Autodesk Inventor part; units mm, degrees
ref_plane "YZ Plane" through (0, 0, 0) normal (1, 0, 0) x (0, 1, 0)
ref_plane "XZ Plane" through (0, 0, 0) normal (0, 1, 0) x (-1, 0, 0)
sketch "Sketch10" plane through (0, 0, 0) normal (0, 1, 0) x (-1, 0, 0)
  line L0 (88.9, 58.7375) -> (-88.9, 58.7375)
  line L1 (-88.9, 58.7375) -> (-88.9, -58.7375)
  line L2 (-88.9, -58.7375) -> (88.9, -58.7375)
  line L3 (88.9, -58.7375) -> (88.9, 58.7375)
  line L4 (88.9, 58.7375) -> (-88.9, -58.7375) construction
  line L5 (-88.9, 58.7375) -> (88.9, -58.7375) construction
  circle A0 centre (0, 0) radius 22.86
  dimension "d56" = 177.8
  dimension "d57" = 45.72
extrude "Extrusion5" add sketch "Sketch10" against normal blind 12.7
sketch "Sketch11" plane through (0, 0, 0) normal (0, 1, 0) x (1, 0, 0)
  point P0 (0, 0)
  point P1 (0, 31.75)
  dimension "d60" = 31.75
hole "Hole4" at (0, 0, -31.75) direction (0, -1, 0) diameter 2.6416 end through all counterbore diameter 4.699 counterbore depth 7.1374
pattern_circular "Circular Pattern1" count 6 over 360 about axis through (0, -10, 0) along (0, 1, 0) of "Hole4"
sketch "Sketch12" plane through (0, 0, 0) normal (0, 1, 0) x (1, 0, 0)
  line L0 (-88.9, -58.7375) -> (-88.9, 58.7375)
  line L1 (-88.9, 58.7375) -> (-38.1, 58.7375)
  line L2 (-38.1, 58.7375) -> (-38.1, 46.0375)
  line L3 (-38.1, 46.0375) -> (-88.9, 46.0375)
  line L4 (-88.9, 46.0375) -> (-88.9, 58.7375)
  point P0 (0, 0)
  dimension "d71" = 12.7
  dimension "d72" = 50.8
extrude "Extrusion6" add sketch "Sketch12" along normal blind 12.7
mirror "Mirror2" about plane through (0, 0, 0) normal (0, 0, 1) of "Extrusion6"
sketch "Sketch13" plane through (88.9, -12.7, -58.7375) normal (0, 0, -1) x (-1, 0, 0)
  line L0 (127, 25.4) -> (177.8, 25.4)
  circle A0 centre (147.6375, 25.4) radius 6.604
  point P0 (88.9, 12.7)
  dimension "d75" = 13.208
extrude "Extrusion7" cut sketch "Sketch13" against normal through all
sketch "Sketch14" plane through (0, 0, 0) normal (0, 1, 0) x (1, 0, 0)
  line L0 (-88.9, 46.0375) -> (-76.2, 46.0375)
  line L1 (-76.2, 46.0375) -> (-76.2, -46.0375)
  line L2 (-76.2, -46.0375) -> (-88.9, -46.0375)
  line L3 (-88.9, -46.0375) -> (-88.9, 46.0375)
  point P0 (0, 0)
  dimension "d78" = 12.7
extrude "Extrusion8" add sketch "Sketch14" along normal blind 25.4
sketch "Sketch15" plane through (0, 0, 0) normal (0, 1, 0) x (1, 0, 0)
  line L0 (88.9, 58.7375) -> (-38.1, 58.7375)
  line L1 (-38.1, -58.7375) -> (88.9, -58.7375)
  line L2 (57.15, 58.7375) -> (69.85, 58.7375)
  line L3 (69.85, 58.7375) -> (69.85, -58.7375)
  line L4 (69.85, -58.7375) -> (57.15, -58.7375)
  line L5 (57.15, -58.7375) -> (57.15, 58.7375)
  line L6 (-88.9, 46.0375) -> (-88.9, -46.0375)
  point P0 (0, 0)
  dimension "d81" = 12.7
  dimension "d82" = 146.05
extrude "Extrusion9" add sketch "Sketch15" along normal blind 25.4
sketch "Sketch16" plane through (0, 0, 0) normal (0, 1, 0) x (1, 0, 0)
  line L0 (88.9, 58.7375) -> (69.85, 58.7375)
  line L1 (88.9, -58.7375) -> (69.85, -58.7375)
  line L2 (69.85, -58.7375) -> (69.85, 58.7375)
  line L3 (69.85, 58.7375) -> (88.9, 58.7375)
  line L4 (88.9, 58.7375) -> (88.9, -58.7375)
  point P0 (0, 0)
extrude "Extrusion10" cut sketch "Sketch16" against normal through all
sketch "Sketch18" plane through (0, -12.7, 0) normal (0, -1, 0) x (1, 0, 0)
  line L0 (-88.9, 58.7375) -> (-88.9, 46.0375) construction
  line L1 (-88.9, 52.3875) -> (69.85, 52.3875) construction
  line L2 (69.85, 58.7375) -> (69.85, -58.7375) construction
  line L3 (-88.9, -58.7375) -> (-88.9, -46.0375) construction
  line L4 (-88.9, -52.3875) -> (69.85, -52.3875) construction
  line L5 (-65.3415, -46.0375) -> (-65.3415, -58.7375)
  line L6 (-65.3415, -58.7375) -> (-88.9, -58.7375)
  line L7 (-88.9, -58.7375) -> (-88.9, -46.0375)
  line L8 (-88.9, -46.0375) -> (-76.2, -46.0375)
  line L9 (-76.2, -46.0375) -> (-65.3415, -46.0375)
  line L10 (-52.1335, -58.7375) -> (-52.1335, -46.0375)
  line L11 (-52.1335, -46.0375) -> (-38.1, -46.0375)
  line L12 (-38.1, -46.0375) -> (-38.1, -58.7375)
  line L13 (-38.1, -58.7375) -> (-52.1335, -58.7375)
  line L14 (-88.9, 58.7375) -> (-88.9, -58.7375)
  line L15 (-88.9, 0) -> (69.85, 0) construction
  line L16 (69.85, -58.7375) -> (69.85, 58.7375) construction
  point P0 (0, 0)
  point P1 (-79.375, -52.3875)
  point P2 (-47.625, -52.3875)
  point P3 (-79.375, 52.3875)
  point P4 (-47.625, 52.3875)
  dimension "d94" = 9.525
  dimension "d95" = 9.525
hole "Hole6" at (-79.375, -12.7, -52.3875) at (-47.625, -12.7, -52.3875) at (-79.375, -12.7, 52.3875) at (-47.625, -12.7, 52.3875) direction (0, 1, 0) diameter 3.81 end through all
sketch "Sketch19" plane through (0, 0, 0) normal (0, 1, 0) x (1, 0, 0)
  line L0 (-74.6125, 31.75) -> (-74.6125, -31.75)
  line L1 (-74.6125, -31.75) -> (-46.0375, -31.75)
  line L2 (-46.0375, -31.75) -> (-46.0375, 31.75)
  line L3 (-46.0375, 31.75) -> (-74.6125, 31.75)
  line L4 (-74.6125, 31.75) -> (-46.0375, -31.75) construction
  line L5 (-74.6125, -31.75) -> (-46.0375, 31.75) construction
  point P0 (0, 0)
  point P1 (-60.325, 0)
extrude "Extrusion11" cut sketch "Sketch19" against normal blind 12.7
equation "\"length\" = 69.0372"
properties part number "SupportForAxel" material "PBT Plastic"
Part model, mm, in its own coordinate system. A direction names the side the tool comes from. Round coordinates to 2 decimals unless told otherwise and drop trailing zeros. Loops run counter-clockwise (first coordinate to the right, second up) from the corner with the lowest first, then second, coordinate; pieces in that order, holes last.
1. 3-axis set-ups, long thin cutter, end or side, ignore diameter. For faces 3 (the face through (-61, -6, 31.75)), 4 (the face through (-77, 12.7, -52)), 5 (the face through (-58.592, 6.098, 52.299)), 6 (the face through (-0.71, -3.62, -29.51)), 7 (the face through (-45, 12.7, 52)): which of +Z, -Z, +X, -X, +Y, -Y reach the whole face in a straight line?
Solutions:
face 3: +Y, -Y
face 4: -Z, -X, +Y
face 5: +Z, -Z, +Y
face 6: +Y
face 7: +Z, -Z, -X, +Y
2. Slice it at B-B (y = 16.5). Give the cut face in (x, z).
Solutions:
outline: (-88.9, -46.04) - (-76.2, -46.04) - (-76.2, 46.04) - (-88.9, 46.04) - close; (57.15, -58.74) - (69.85, -58.74) - (69.85, 58.74) - (57.15, 58.74) - close
3. Slice it at C-C (x = -70). Give the cut face in (y, z), and give its area (3 significant figures).
Solutions:
outline: (-12.7, -58.74) - (12.7, -58.74) - (12.7, -46.04) - (0, -46.04) - (0, -31.75) - (-12.7, -31.75) - close; (-12.7, 31.75) - (0, 31.75) - (0, 46.04) - (12.7, 46.04) - (12.7, 58.74) - (-12.7, 58.74) - close
area: 1,010 mm2
4. Flat gauge pins, fed straight in: pin 1 (6 mm diameter, centred on x = -47.62, z = 52.39, fed in from +Y); pin 2 (7.5 mm diameter, centred on x = 27.5, z = 15.88, fed in from +Y); pin 3 (3 mm diameter, centred on x = 0, z = -31.75, fed in from +Y). Where does each tip first touch, or does it go through?
Solutions:
pin 1: stops at y = 12.7
pin 2: stops at y = 0
pin 3: stops at y = -7.14
5. Two-plate mould, pull along Z, no slides. Class faces 1 (the face through (57.15, 13, 1)), 2 (the face through (-46.038, -6, 0)): pulls with the +Z half, pulls with the -Z half, needs draft (parallel to the pull), parting line crosses it, or undercut.
Solutions:
face 1: needs draft
face 2: undercut
6. Slice it at A-A (z = 0). Give the cut face in (x, y), and give its area (3 significant figures).
Solutions:
outline: (-88.9, -12.7) - (-74.61, -12.7) - (-74.61, 0) - (-76.2, 0) - (-76.2, 25.4) - (-88.9, 25.4) - close; (-46.04, -12.7) - (-22.86, -12.7) - (-22.86, 0) - (-46.04, 0) - close; (22.86, -12.7) - (69.85, -12.7) - (69.85, 25.4) - (57.15, 25.4) - (57.15, 0) - (22.86, 0) - close
area: 1,720 mm2
7. Slice it at D-D (y = -5). Count the separate pieces of the cut face and the enclosed holes in it, and give its area (3 significant figures).
Solutions:
separate pieces: 1
enclosed holes: 12
area: 15,000 mm2
8. Drill centre lines: line 1 along X through (y, z) = (17.5, 8); line 2 along Z through (x, y) = (-67, -7.5); line 3 along X through (y, z) = (-9, 23). Where is each one in solid material? Low to high.
Solutions:
line 1: x = -88.9 to -76.2, 57.15 to 69.85
line 2: z = -58.74 to -31.75, 31.75 to 58.74
line 3: x = -88.9 to -74.61, -46.04 to 69.85
